The figure shows three views and two pictorial views of one solid part (mm, origin at its lowest corner). Answer the questions. A direction names the side the tool comes from. Coordinates: 2 decimals unless noted, no trailing zeros. Write each loop counter-clockwise with the first axis right and the second up, starting at its lowest first coordinate (ties: lowest second). Pieces come first, ordered by that corner, then holes.
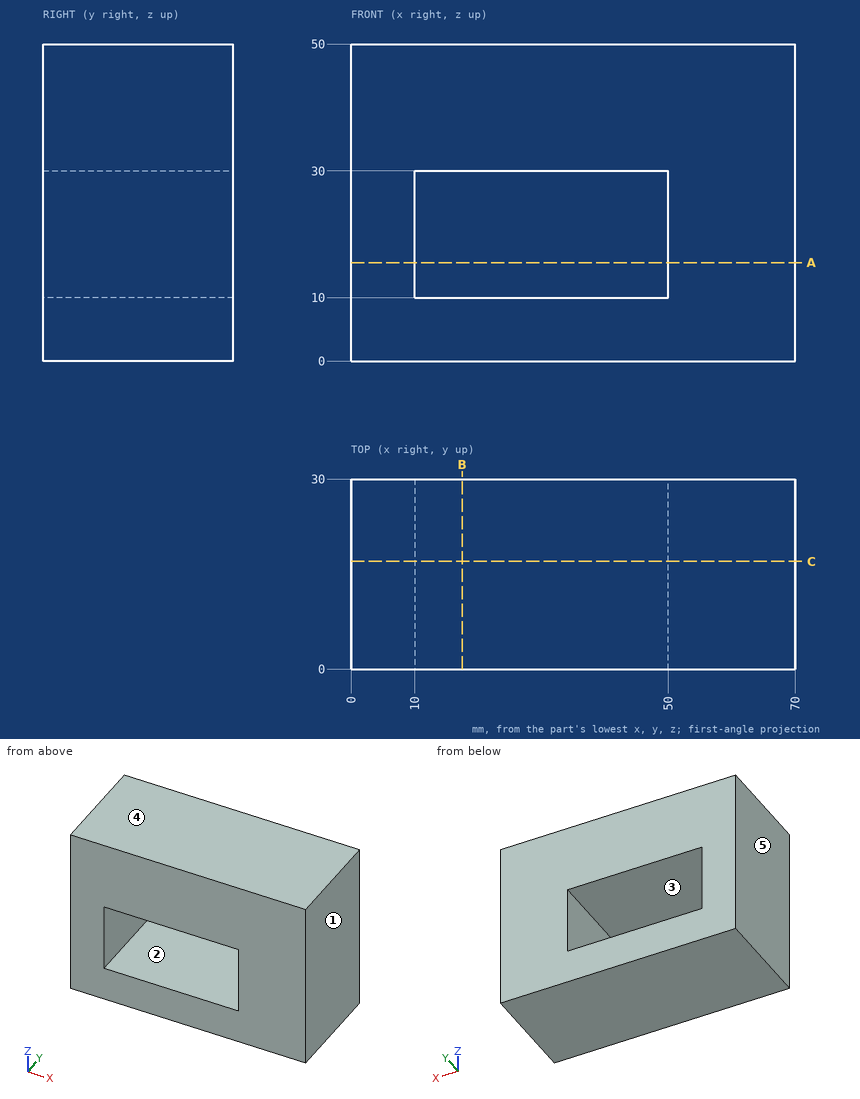
Q1. Which of the six approach directions +Z, -Z, +X, -X, +Y, -Y give full straight-line access (tool end or side, diameter ignored) to the marked faces 1 and 2?
Answers below:
face 1: +Z, -Z, +X, +Y, -Y
face 2: +Y, -Y
Q2. Given pin 1 (3 mm diameter, centred on x = 9.5, y = 21, fed in from -Z), flat-ended and moving along its own axis, determine where the tip first touches the part or whether it passes through.
Answers below:
pin 1: stops at z = 0
Q3. The part is cut by section B-B, the plane x = 17.5. Write down the section's boundary in (y, z).
Answers below:
outline: (0, 0) - (30, 0) - (30, 10) - (0, 10) - close; (0, 30) - (30, 30) - (30, 50) - (0, 50) - close
Q4. Find the intervals of material crossed by probe 1 along X at (y, z) = (14.5, 17.5); probe 2 along Z at (x, y) = (42, 9.25), in increasing order.
Answers below:
probe 1: x = 0 to 10, 50 to 70
probe 2: z = 0 to 10, 30 to 50
Q5. Determine the mould class of the marked faces 3, 4 and 5 for opening direction Z: released by +Z, released by -Z, zero draft, split by the parting line, or undercut.
Answers below:
face 3: undercut
face 4: released by +Z
face 5: zero draft
Q6. The part is cut by section C-C, the plane y = 17. Write down the section's boundary in (x, z).
Answers below:
outline: (0, 0) - (70, 0) - (70, 50) - (0, 50) - close; hole (10, 10) - (50, 10) - (50, 30) - (10, 30) - close
Q7. The part is cut by section A-A, the plane z = 15.5. Write down the section's boundary in (x, y), then the cut area to 3 significant figures.
Answers below:
outline: (0, 0) - (10, 0) - (10, 30) - (0, 30) - close; (50, 0) - (70, 0) - (70, 30) - (50, 30) - close
area: 900 mm2
